For this review, take the finished solid that the model builds, in its own axes (mm). Give positions to 0.01 mm unless a question says otherwise; leave off trailing zeros. Write each loop counter-clockwise with the first axis right and the second up, starting at its lowest first coordinate (ties: lowest second). Pieces come first, ordered by that corner, then holes.
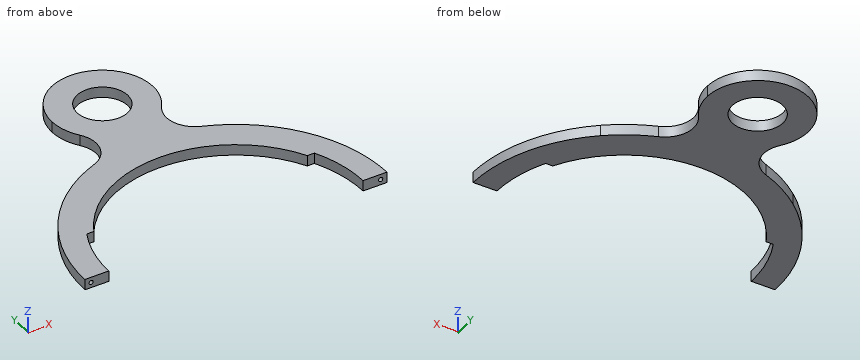
from build123d import *
from build123d.topology import SkipClean

# Parameters (mm, degrees)
SKETCH_1_R             = 20
EXTRUDE_1_DEPTH        = 8.5
HOLE_WIZARD_M4_1_D     = 3.3
HOLE_WIZARD_M4_1_DEPTH = 10.1
HOLE_WIZARD_M4_1_TIP   = 0.991420021
CUT_EXTRUDE_START      = -10
CUT_EXTRUDE_1_DEPTH    = 10


with BuildPart() as part:
    # 草图1 → 凸台-拉伸1 (new body)
    with BuildSketch(Plane.XY):
        with BuildLine():
            Line((-40, 170), (-40, 169.705627485))
            ThreePointArc((-40, 169.705627485), (-49.546596627, 127.065484214), (-76.363636364, 92.566705901))
            ThreePointArc((-76.363636364, 92.566705901), (-108.544084048, 51.168171925), (-120, 0))
            Line((-120, 0), (-101, 0))
            ThreePointArc((-101, 0), (-98.319745933, 23.113363226), (-90.421236444, 45))
            Line((-90.421236444, 45), (-84.799764151, 45))
            ThreePointArc((-84.799764151, 45), (0, 96), (84.799764151, 45))
            Line((84.799764151, 45), (90.421236444, 45))
            ThreePointArc((90.421236444, 45), (98.319745933, 23.113363226), (101, 0))
            Line((101, 0), (120, 0))
            ThreePointArc((120, 0), (108.544084048, 51.168171925), (76.363636364, 92.566705901))
            ThreePointArc((76.363636364, 92.566705901), (49.546596627, 127.065484214), (40, 169.705627485))
            Line((40, 169.705627485), (40, 170))
            ThreePointArc((40, 170), (0, 210), (-40, 170))
        make_face()
        with Locations((0, 170)):
            Circle(SKETCH_1_R, mode=Mode.SUBTRACT)
    extrude(amount=EXTRUDE_1_DEPTH)

    # M4 螺纹孔1
    with Locations(Plane(origin=(-115, 0, 4.25), x_dir=(0, 0, -1), z_dir=(0, -1, 0))):
        with Locations((0, 0), (0, 230)):
            Hole(HOLE_WIZARD_M4_1_D / 2, depth=HOLE_WIZARD_M4_1_DEPTH)
            with Locations((0, 0, -(HOLE_WIZARD_M4_1_DEPTH + HOLE_WIZARD_M4_1_TIP / 2))):  # 118° drill point
                Cone(0, HOLE_WIZARD_M4_1_D / 2, HOLE_WIZARD_M4_1_TIP, mode=Mode.SUBTRACT)

    # 草图5 → 切除-拉伸1 (cut)
    with SkipClean():  # the faces are left unmerged after this step: merging them gives an invalid solid
        with BuildSketch(Plane.XY.offset(8.5).offset(CUT_EXTRUDE_START)):
            with BuildLine():
                Line((-40, 170), (-40, 169.705627485))
                ThreePointArc((-40, 169.705627485), (-49.546596627, 127.065484214), (-76.363636364, 92.566705901))
                ThreePointArc((-76.363636364, 92.566705901), (-60.26783628, 103.76795223), (-42.562622554, 112.198142415))
                ThreePointArc((-42.562622554, 112.198142415), (-28.980506646, 126.808479049), (-32.347593141, 146.470588235))
                ThreePointArc((-32.347593141, 146.470588235), (-38.038820471, 157.628737446), (-40, 170))
            make_face()
        cut_extrude_1 = extrude(amount=CUT_EXTRUDE_1_DEPTH, mode=Mode.SUBTRACT)

    # 镜向1: 切除-拉伸1 across plane
    with SkipClean():  # the faces are left unmerged after this step: merging them gives an invalid solid
        add(cut_extrude_1.mirror(Plane(origin=(0, 0, 0), x_dir=(0, 0, 1), z_dir=(1, 0, 0))), mode=Mode.SUBTRACT)


solid = part.part
(1) For L1, parallel to X at y = 2.5, z = 4.25; L2, parallel to Y at x = -1, z = 6.25; L3, parallel to Z at x = -115, y = 4.5, list the stretches that pass through material, from the lowest coordinate up.
(2) We need section C-C (y = 193). Write out the cut boundary in (x, z), and give its area (3 significant figures).
(3) We need section B-B (y = 35.5). Write out the cut boundary in (x, z), and give its area (3 significant figures).
(4) We need section A-A (x = 0). Write out the cut boundary in (y, z).
(5) Clearance check with flat-ended pins moving along their axes: pin 1 Ø3 at (x, z) = (88, 4) entering from -Y; pin 2 Ø1.5 at (x, z) = (13.5, 5) entering from -Y; pin 3 Ø1 at (y, z) = (47.5, 3.5) entering from +X. State where each tip first meets the part, or that it passes through.
The answers:
1. L1: x = -119.97 to -116.65, -113.35 to -100.97, 100.97 to 113.35, 116.65 to 119.97
1. L2: y = 95.99 to 150.03, 189.97 to 209.99
1. L3: z = 0 to 2.6, 5.9 to 8.5
2. outline: (-32.73, 0) - (32.73, 0) - (32.73, 8.5) - (-32.73, 8.5) - close
2. area: 556 mm2
3. outline: (-114.63, 0) - (-94.56, 0) - (-94.56, 8.5) - (-114.63, 8.5) - close; (94.56, 0) - (114.63, 0) - (114.63, 8.5) - (94.56, 8.5) - close
3. area: 341 mm2
4. outline: (96, 0) - (150, 0) - (150, 8.5) - (96, 8.5) - close; (190, 0) - (210, 0) - (210, 8.5) - (190, 8.5) - close
5. pin 1: stops at y = 45
5. pin 2: stops at y = 94.94
5. pin 3: stops at x = 110.41
